from build123d import *
from build123d.topology import SkipClean

# Parameters (mm, degrees)
SKETCH1_R             = 3.3734375
BOSS_EXTRUDE1_DEPTH   = 6
BOSS_EXTRUDE1_2_DEPTH = 6
BOSS_EXTRUDE2_START   = 2
SKETCH2_R             = 3.3734375
BOSS_EXTRUDE2_DEPTH   = 2
SKETCH3_R             = 10.5
BOSS_EXTRUDE3_DEPTH   = 2
BOSS_EXTRUDE4_START   = 2
SKETCH4_R             = 10.5
BOSS_EXTRUDE4_DEPTH   = 2
BOSS_EXTRUDE5_START   = 6
SKETCH5_R             = 10.5
SKETCH5_R_2           = 1.5
BOSS_EXTRUDE5_DEPTH   = 6
FILLET1_R             = 7
SKETCH6_W             = 15
SKETCH6_H             = 15
SKETCH6_R             = 3.3734375
BOSS_EXTRUDE6_DEPTH   = 12
SKETCH7_R             = 5.5
CUT_EXTRUDE2_DEPTH    = 15
SKETCH8_W             = 8
SKETCH8_H             = 15
CUT_EXTRUDE3_DEPTH    = 5.2
SKETCH9_W             = 8
SKETCH9_H             = 15
CUT_EXTRUDE4_DEPTH    = 5.2
FILLET2_R             = 7.5


# Some blends are built 0.0001 mm under size
with BuildPart() as part:
    # Sketch1 → Boss-Extrude1 (new body)
    with BuildSketch(Plane.XY):
        with BuildLine():
            ThreePointArc((11.5, 0), (10.782037741, -3.999707758), (8.717797887, -7.5))
            Line((8.717797887, -7.5), (38.1, -7.5))
            Line((38.1, -7.5), (38.1, 7.5))
            Line((38.1, 7.5), (8.717797887, 7.5))
            ThreePointArc((8.717797887, 7.5), (10.782037741, 3.999707758), (11.5, 0))
        make_face()
        with Locations((25.4, 0)):
            Circle(SKETCH1_R, mode=Mode.SUBTRACT)
    extrude(amount=BOSS_EXTRUDE1_DEPTH)



with BuildPart() as body_2:
    # Sketch1 → Boss-Extrude1 2 (new body)
    with BuildSketch(Plane.XY):
        with BuildLine():
            Line((-38.1, 7.5), (-38.1, -7.5))
            Line((-38.1, -7.5), (-8.717797887, -7.5))
            ThreePointArc((-8.717797887, -7.5), (-11.5, 0), (-8.717797887, 7.5))
            Line((-8.717797887, 7.5), (-38.1, 7.5))
        make_face()
        with Locations((-25.4, 0)):
            Circle(SKETCH1_R, mode=Mode.SUBTRACT)
    extrude(amount=BOSS_EXTRUDE1_2_DEPTH)


with BuildPart() as part_1:
    with SkipClean():  # the faces are left unmerged after this step: merging them gives an invalid solid
        add(part.part)

        add(body_2.part)  # Boss-Extrude2 merges body 2
        # Sketch2 → Boss-Extrude2 (add)
        # profile 1 of 3: a face of its own
        with BuildSketch(Plane(origin=(0, 0, 0), x_dir=(-1, 0, 0), z_dir=(0, 0, -1)).offset(BOSS_EXTRUDE2_START)):
            with BuildLine():
                Line((-38.1, -7.5), (-8.717797887, -7.5))
                ThreePointArc((-8.717797887, -7.5), (-11.5, 0), (-8.717797887, 7.5))
                Line((-8.717797887, 7.5), (-38.1, 7.5))
                Line((-38.1, 7.5), (-38.1, -7.5))
            make_face()
            with Locations((-25.4, 0)):
                Circle(SKETCH2_R, mode=Mode.SUBTRACT)
        # profile 2 of 3: a face of its own
        with BuildSketch(Plane(origin=(0, 0, 0), x_dir=(-1, 0, 0), z_dir=(0, 0, -1)).offset(BOSS_EXTRUDE2_START)):
            with BuildLine():
                Line((-8.717797887, -7.5), (8.717797887, -7.5))
                ThreePointArc((8.717797887, -7.5), (11.5, 0), (8.717797887, 7.5))
                Line((8.717797887, 7.5), (-8.717797887, 7.5))
                ThreePointArc((-8.717797887, 7.5), (-11.5, 0), (-8.717797887, -7.5))
            make_face()
        # profile 3 of 3: a face of its own
        with BuildSketch(Plane(origin=(0, 0, 0), x_dir=(-1, 0, 0), z_dir=(0, 0, -1)).offset(BOSS_EXTRUDE2_START)):
            with BuildLine():
                ThreePointArc((8.717797887, -7.5), (11.5, 0), (8.717797887, 7.5))
                Line((8.717797887, 7.5), (38.1, 7.5))
                Line((38.1, 7.5), (38.1, -7.5))
                Line((38.1, -7.5), (8.717797887, -7.5))
            make_face()
            with Locations(Location((25.4, 0, 0), (0, 0, 180))):
                Circle(SKETCH2_R, mode=Mode.SUBTRACT)
        extrude(amount=-BOSS_EXTRUDE2_DEPTH)

    # Sketch3 → Boss-Extrude3 (add)
    with SkipClean():  # the faces are left unmerged after this step: merging them gives an invalid solid
        with BuildSketch(Plane(origin=(0, 0, -2), x_dir=(-1, 0, 0), z_dir=(0, 0, -1))):
            Circle(SKETCH3_R)
        extrude(amount=-BOSS_EXTRUDE3_DEPTH)

    # Sketch4 → Boss-Extrude4 (add)
    with SkipClean():  # the faces are left unmerged after this step: merging them gives an invalid solid
        with BuildSketch(Plane(origin=(0, 0, -2), x_dir=(-1, 0, 0), z_dir=(0, 0, -1)).offset(BOSS_EXTRUDE4_START)):
            Circle(SKETCH4_R)
        extrude(amount=-BOSS_EXTRUDE4_DEPTH)

    # Sketch5 → Boss-Extrude5 (add)
    with SkipClean():  # the faces are left unmerged after this step: merging them gives an invalid solid
        with BuildSketch(Plane(origin=(0, 0, -4), x_dir=(-1, 0, 0), z_dir=(0, 0, -1)).offset(BOSS_EXTRUDE5_START)):
            Circle(SKETCH5_R)
            Circle(SKETCH5_R_2, mode=Mode.SUBTRACT)
        extrude(amount=-BOSS_EXTRUDE5_DEPTH)

    # Fillet1
    # the kernel refuses this fillet: 7 mm, written as the material it adds along each edge
    with BuildSketch(Plane(origin=(0, 0, -2), x_dir=(-1, 0, 0), z_dir=(0, -1, 0))) as fillet1_piece_1_section:
        with BuildLine():
            CenterArc((10.5 + FILLET1_R, FILLET1_R), FILLET1_R, 180, 90)
            Line((10.5 + FILLET1_R, 0), (10.5, 0))
            Line((10.5, 0), (10.5, FILLET1_R))
        make_face()
    fillet1_piece_1 = revolve(axis=Axis((0, 0, -2), (0, 0, -1)), revolution_arc=141.087496106, mode=Mode.PRIVATE)
    fillet1_piece_1 = split(fillet1_piece_1, bisect_by=Plane(origin=(-11.14561096, 7.5, -3.604307229), z_dir=(0, -1, 0)), keep=Keep.TOP, mode=Mode.PRIVATE)
    add(fillet1_piece_1)
    with BuildSketch(Plane(origin=(0, 0, -2), x_dir=(-0.7784296665775441, 0.627731833024241, 0), z_dir=(-0.627731833024241, -0.7784296665775441, 0))) as fillet1_piece_2_section:
        with BuildLine():
            CenterArc((10.5 + FILLET1_R, FILLET1_R), FILLET1_R, 180, 90)
            Line((10.5, FILLET1_R), (10.5, 0))
            Line((10.5, 0), (10.5 + FILLET1_R, 0))
        make_face()
    fillet1_piece_2 = revolve(axis=Axis((0, 0, -2), (0, 0, -1)), revolution_arc=282.234042337, mode=Mode.PRIVATE)
    fillet1_piece_2 = split(fillet1_piece_2, bisect_by=Plane(origin=(-8.090689078, 7.5, -4.608700721), z_dir=(0, -1, 0)), keep=Keep.TOP, mode=Mode.PRIVATE)
    fillet1_piece_2 = split(fillet1_piece_2, bisect_by=Plane(origin=(-8.090689078, -7.5, -4.608700721), z_dir=(0, 1, 0)), keep=Keep.TOP, mode=Mode.PRIVATE)
    add(fillet1_piece_2)
    with BuildSketch(Plane(origin=(0, 0, -2), x_dir=(0.7781060870335762, -0.6281328818978487, 0), z_dir=(0.6281328818978487, 0.7781060870335762, 0))) as fillet1_piece_3_section:
        with BuildLine():
            CenterArc((10.5 + FILLET1_R, FILLET1_R), FILLET1_R, 180, 90)
            Line((10.5 + FILLET1_R, 0), (10.5, 0))
            Line((10.5, 0), (10.5, FILLET1_R))
        make_face()
    fillet1_piece_3 = revolve(axis=Axis((0, 0, -2), (0, 0, -1)), revolution_arc=141.087496106, mode=Mode.PRIVATE)
    fillet1_piece_3 = split(fillet1_piece_3, bisect_by=Plane(origin=(8.086917583, -7.5, -4.611323589), z_dir=(0, 1, 0)), keep=Keep.TOP, mode=Mode.PRIVATE)
    add(fillet1_piece_3)

    # Sketch6 → Boss-Extrude6 (add)
    with BuildSketch(Plane.XY.offset(6)):
        with Locations((25.4, 0)):
            Rectangle(SKETCH6_W, SKETCH6_H)
        with Locations(Location((25.4, 0, 0), (0, 0, 180))):
            Circle(SKETCH6_R, mode=Mode.SUBTRACT)
    boss_extrude6 = extrude(amount=BOSS_EXTRUDE6_DEPTH)

    # Sketch7 → Cut-Extrude2 (cut)
    with BuildSketch(Plane(origin=(0, 0, -2), x_dir=(-1, 0, 0), z_dir=(0, 0, -1))):
        with Locations((-25.4, 0)):
            Circle(SKETCH7_R)
    cut_extrude2 = extrude(amount=-CUT_EXTRUDE2_DEPTH, mode=Mode.SUBTRACT)

    # Sketch8 → Cut-Extrude3 (cut)
    with BuildSketch(Plane(origin=(38.1, 0, 0), x_dir=(0, 0, -1), z_dir=(1, 0, 0))):
        with Locations((-2, 0)):
            Rectangle(SKETCH8_W, SKETCH8_H)
    extrude(amount=-CUT_EXTRUDE3_DEPTH, mode=Mode.SUBTRACT)

    # Mirror1: Boss-Extrude6, Cut-Extrude2 across plane
    add(boss_extrude6.mirror(Plane(origin=(0, 0, 0), x_dir=(0, 0, 1), z_dir=(1, 0, 0))))
    add(cut_extrude2.mirror(Plane(origin=(0, 0, 0), x_dir=(0, 0, 1), z_dir=(1, 0, 0))), mode=Mode.SUBTRACT)

    # Sketch9 → Cut-Extrude4 (cut)
    with BuildSketch(Plane.ZY.offset(38.1)):
        with Locations((2, 0)):
            Rectangle(SKETCH9_W, SKETCH9_H)
    extrude(amount=-CUT_EXTRUDE4_DEPTH, mode=Mode.SUBTRACT)

    # Fillet2
    fillet2_edges = [part_1.edges().sort_by_distance(p)[0] for p in [
        (32.9, -7.5, 8),
        (32.9, 7.5, 8),
        (-32.9, 7.5, 8),
        (-32.9, -7.5, 8),
    ]]
    fillet(fillet2_edges, radius=FILLET2_R - 0.0001)  # a hair under: the kernel refuses the full size


solid = part_1.part
For this review, take the finished solid that the model builds, in its own axes (mm). A direction names the side the tool comes from. Round coordinates to 2 decimals unless told otherwise and drop trailing zeros. Order: outer loops, then holes, each group sorted by start corner. A loop starts at its lowest first (then second) coordinate and runs counter-clockwise, first axis right, second up. Notation, with made-up numbers: (44, 60) -> (65, 60) arc R17 cw to (65, 66) -> close; hole circle Ø5 at (3.5, 85.5). An arc over 180 degrees is marked (long way). Put each result on its own line as item: value.
Q1. Machinability: for faces 1 (the cylindrical face through (1.5, 0.07, -7.04)), 2 (the flat face through (-18, 7.5, 4)), 3 (the cylindrical face through (-11.5, -0.1, 3)), which of the approach directions +Z, -Z, +X, -X, +Y, -Y give a long, thin tool a straight path to every point of the face, cutting with its end or side? Answer none if there is none.
Check result:
face 1: -Z
face 2: +Z, -Z, -X, +Y
face 3: +Z
Q2. Insertion check: pin 1 Ø9 at (x, z) = (-19, 4.5) entering from -Y; pin 2 Ø12 at (x, z) = (4.5, 5.5) entering from -Y; pin 3 Ø4.5 at (x, y) = (-26, -3) entering from -Z; pin 4 Ø6.5 at (x, y) = (-25.4, 0) entering from -Z. Each pin has a flat end and moves straight along its axis. Give the tip position at first contact, or say it passes through.
Check result:
pin 1: y = -7.5
pin 2: y = -10.29
pin 3: z = 13
pin 4: through
Q3. Mouldability with a two-part tool opening along Y and no side actions: class faces 4 (the flat face through (18, -7.5, 4)), 5 (the cylindrical face through (-5.645, 8.854, -5.07)), 6 (the cylindrical face through (-30.895, 0.242, 5.395)) as pulls with the +Y half, pulls with the -Y half, needs draft (parallel to the pull), parting line crosses it, or undercut.
Check result:
face 4: pulls with the -Y half
face 5: parting line crosses it
face 6: undercut
Q4. Add section A-A on z = 4.5. State how many separate pieces and enclosed holes the cut face has, plus the area to 3 significant figures.
Check result:
separate pieces: 2
enclosed holes: 2
area: 430 mm2
Q5. Add section B-B on x = 0. Write out the cut boundary in (y, z), plus the area to 3 significant figures.
Check result:
outline: (-10.5, -10) -> (-1.5, -10) -> (-1.5, -4) -> (1.5, -4) -> (1.5, -10) -> (10.5, -10) -> (10.5, 0) -> (-10.5, 0) -> close
area: 192 mm2
Q6. For probe 1 along X at (y, z) = (-2, 0.75); probe 2 along X at (y, z) = (2.25, 15.75); probe 3 along Y at (x, z) = (25.4, 14.1), list the stretches that pass through material, from the lowest coordinate up. Write a range as [from, to].
Check result:
probe 1: [-32.63, -30.52], [-20.28, -11.32], [11.32, 20.28], [30.52, 32.63]
probe 2: [-32.55, -27.91], [-22.89, -17.9], [17.9, 22.89], [27.91, 32.55]
probe 3: [-7.5, -3.37], [3.37, 7.5]
